For this review, use the dimensioned drawing (mm, ordinates from the lowest corner) and the shaded views. A direction names the side the tool comes from. Coordinates: 2 decimals unless noted, no trailing zeros. Write each loop counter-clockwise with the first axis right and the second up, starting at its lowest first coordinate (ties: lowest second). Pieces come first, ordered by that corner, then holes. Notation, with made-up numbers: (-15.5, 2) -> (19.5, 2) arc R21 cw to (19.5, 16) -> close; hole circle Ø8 at (-17.5, -5). An arc over 180 degrees is marked (long way). Put each result on its own line as item: value. Start each with the question number.
Item 1: To check wall thickness, follow L1, parallel to X at y = 12.7, z = 19.75; L2, parallel to Y at x = 25.4, z = 6; L3, parallel to Z at x = 41.75, y = 12.7. State the ranges of each line that lie inside material, in increasing order.
Item 2: The part is to be moulded in two halves that separate along Z. For the marked faces 1, 2, 3 and 4, say which applies: +Z half, -Z half, draft (parallel to the pull), parting line (faces both ways), or undercut.
Item 3: Consider section A-A on x = 18.5. Give the boundary of the cut face in (y, z), and give its area (3 significant figures).
Item 4: For the marked faces 5, 6 and 7, list the 3-axis set-ups (+Z, -Z, +X, -X, +Y, -Y) from which the entire face can be reached by the end or side of a thin tool; tool diameter is ignored.
Item 5: Insertion check: P1, Ø6.5, axis at x = 12.7, y = 12.7, coming from the +Z side; P2, Ø6, axis at y = 11.5, z = 6, coming from the -X side; P3, Ø6, axis at y = 12.7, z = 12.7, coming from the +X side. Each pin has a flat end and moves straight along its axis. Give the tip position at first contact, or say it passes through.
Item 6: Consider section B-B on y = 12.7. Give the number of separate pieces and of enclosed holes in the cut face, and give its area (3 significant figures).
Item 7: Consider section D-D on z = 24. Give the boundary of the cut face in (x, y), and give its area (3 significant figures).
Item 8: Consider section C-C on y = 18. Give the boundary of the cut face in (x, z), and give its area (3 significant figures).
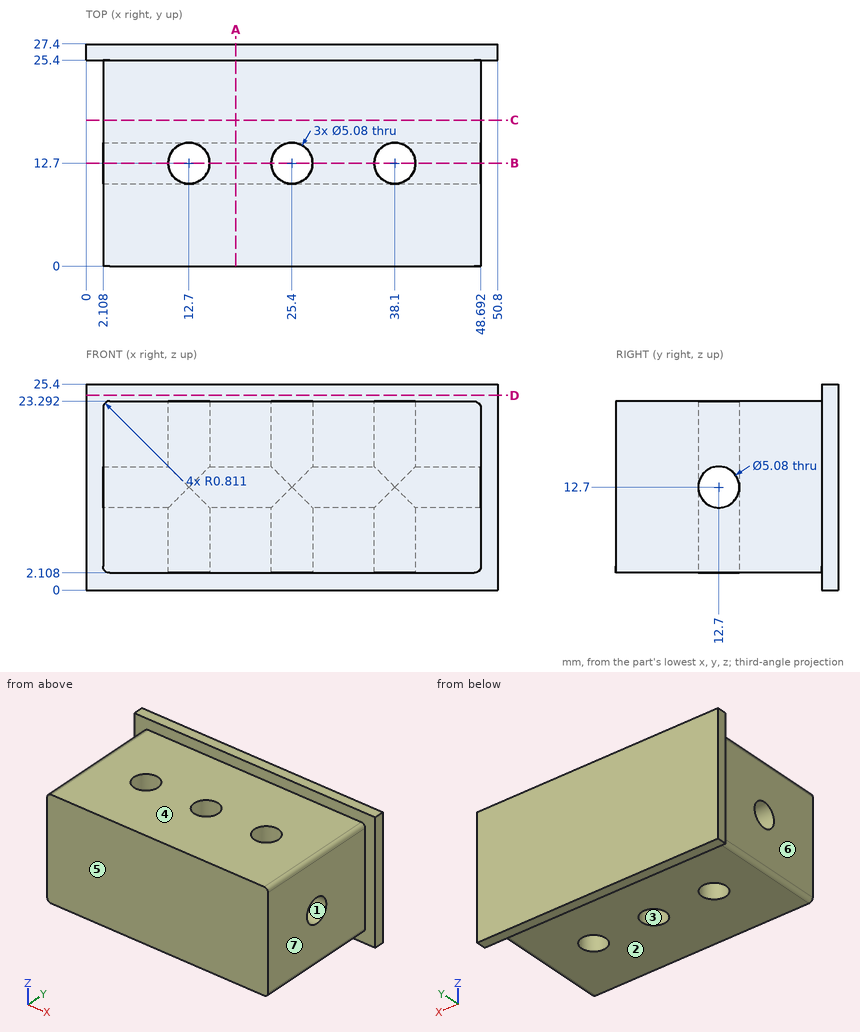
Return value:
1. L1: 2.11 to 10.16, 15.24 to 22.86, 27.94 to 35.56, 40.64 to 48.69
1. L2: 0 to 10.16, 15.24 to 27.4
1. L3: 2.11 to 10.16, 15.24 to 23.29
2. face 1: undercut
2. face 2: -Z half
2. face 3: draft
2. face 4: +Z half
3. outline: (0, 2.11) -> (25.4, 2.11) -> (25.4, 0) -> (27.4, 0) -> (27.4, 25.4) -> (25.4, 25.4) -> (25.4, 23.29) -> (0, 23.29) -> close; hole circle Ø5.08 at (12.7, 12.7)
3. area: 569 mm^2
4. face 5: +Z, -Z, +X, -X, -Y
4. face 6: +Z, -Z, -X, -Y
4. face 7: +Z, -Z, +X, -Y
5. P1: z = 23.29
5. P2: x = 2.11
5. P3: x = 48.69
6. separate pieces: 8
6. enclosed holes: 0
6. area: 504 mm^2
7. outline: (0, 25.4) -> (50.8, 25.4) -> (50.8, 27.4) -> (0, 27.4) -> close
7. area: 102 mm^2
8. outline: (2.11, 2.92) arc R0.81 ccw to (2.92, 2.11) -> (47.88, 2.11) arc R0.81 ccw to (48.69, 2.92) -> (48.69, 22.48) arc R0.81 ccw to (47.88, 23.29) -> (2.92, 23.29) arc R0.81 ccw to (2.11, 22.48) -> close
8. area: 986 mm^2
